Check sheet for the modelled part. Datum: model origin and axes. Units: mm. Round coordinates to 2 decimals unless told otherwise and drop trailing zeros. Loops run counter-clockwise (first coordinate to the right, second up) from the corner with the lowest first, then second, coordinate; pieces in that order, holes last. Notation, with made-up numbers: (-24.75, 42) -> (4.25, 42) arc R18 cw to (4.25, 61) -> close; hole circle Ø9 at (21, -9). An arc over 180 degrees is marked (long way). Return JSON: item names as keys, results as strings.
Autodesk Inventor part; units mm, degrees
ref_plane "YZ Plane" through (0, 0, 0) normal (1, 0, 0) x (0, 1, 0)
ref_plane "XZ Plane" through (0, 0, 0) normal (0, 1, 0) x (-1, 0, 0)
ref_plane "XY Plane" through (0, 0, 0) normal (0, 0, 1) x (1, 0, 0)
sketch "スケッチ3" plane through (0, 0, 0) normal (0, 0, 1) x (1, 0, 0)
  line L0 (60, -99.3436) -> (-60, -99.3436)
  line L1 (-60, -99.3436) -> (-60, 99.3436)
  line L2 (-60, 99.3436) -> (60, 99.3436)
  line L3 (60, 99.3436) -> (60, -99.3436)
  line L4 (60, -99.3436) -> (-60, 99.3436) construction
  line L5 (-60, -99.3436) -> (60, 99.3436) construction
  point P0 (0, 0)
  dimension "d25" = 120
extrude "押し出し1" add sketch "スケッチ3" against normal blind 3
sketch "スケッチ4" plane through (0, 0, 0) normal (0, 0, 1) x (1, 0, 0)
  line L0 (0, 45.0711) -> (68.3595, 45.0711)
  line L1 (68.3595, 45.0711) -> (-74.3824, 45.0711)
  line L2 (-74.3824, 45.0711) -> (108.1656, 45.0711)
  line L3 (108.1656, 45.0711) -> (108.1656, 129.4154)
  line L4 (108.1656, 129.4154) -> (-74.3824, 129.4154)
  line L5 (-74.3824, 129.4154) -> (-74.3824, 45.0711)
  point P0 (0, 0)
extrude "押し出し4" cut sketch "スケッチ4" against normal blind 10
sketch "スケッチ12" plane through (0, 0, 0) normal (0, 0, 1) x (1, 0, 0)
  circle A0 centre (0, 0) radius 9
  circle A1 centre (0, 0) radius 22.5
  dimension "d85" = 18
  dimension "d93" = 45
sketch "スケッチ13" plane through (0, 0, 0) normal (0, 0, 1) x (1, 0, 0)
  circle A0 centre (0, 0) radius 7.5
  circle A1 centre (0, 0) radius 32.5
  circle A2 centre (31.7707, 6.8465) radius 25
  circle A3 centre (31.7707, 6.8465) radius 7.5
  circle A4 centre (31.7707, 6.8465) radius 32.5
  circle A5 centre (28.5436, -25.4929) radius 25
  circle A6 centre (28.5436, -25.4929) radius 20
  circle A7 centre (28.5436, -25.4929) radius 60
  circle A8 centre (0, -78.2685) radius 40
  circle A9 centre (0, -78.2685) radius 50
  circle A10 centre (31.7707, 6.8465) radius 5.05
  circle A11 centre (28.5436, -25.4929) radius 9.55
  circle A12 centre (0, -78.2685) radius 9.55
  dimension "d87" = 65
  dimension "d89" = 65
  dimension "d91" = 120
  dimension "d86" = 15
  dimension "d88" = 15
  dimension "d90" = 40
  dimension "d92" = 100
  dimension "d96" = 10.1
  dimension "d97" = 19.1
  dimension "d98" = 19.1
extrude "押し出し15" cut sketch "スケッチ12" against normal blind 10 contours A0
extrude "押し出し16" cut sketch "スケッチ13" against normal blind 10 contours A10 A1 | A1 A10 | A11 A1 A2 | A2 A1 A4 A11 | A4 A1 A11 | A2 A11 A4 A1 | A1 A11 A2 | A4 A11 A1 | A12 A7 | A7 A12
sketch "スケッチ14" plane through (0, 0, 0) normal (0, 0, 1) x (1, 0, 0)
  line L0 (-60, -99.3436) -> (-60, 45.0711)
  line L1 (60, 45.0711) -> (60, -99.3436)
  line L2 (-60, 45.0711) -> (60, 45.0711)
  line L3 (60, 45.0711) -> (60, -92.9289)
  line L4 (60, -92.9289) -> (-60, -92.9289)
  line L5 (-60, -92.9289) -> (-60, 45.0711)
  point P0 (0, 0)
  dimension "d101" = 138
extrude "押し出し17" cut sketch "スケッチ14" against normal blind 10 keep common part
sketch "スケッチ15" plane through (-60, 45.0711, 0) normal (0, 1, 0) x (1, 0, 0)
  line L0 (-15.5399, 21.7204) -> (138.9638, 21.7204)
  line L1 (138.9638, 21.7204) -> (138.9638, -41.1938)
  line L2 (138.9638, -41.1938) -> (-15.5399, -41.1938)
  line L3 (-15.5399, -41.1938) -> (-15.5399, 21.7204)
  point P0 (60, 0)
extrude "押し出し18" cut sketch "スケッチ15" against normal blind 10
sketch "スケッチ16" plane through (0, 0, 0) normal (0, 0, 1) x (1, 0, 0)
  circle A0 centre (31.7707, 6.8465) radius 5.05
  circle A1 centre (31.7707, 6.8465) radius 25
  circle A2 centre (28.5436, -25.4929) radius 9.55
  circle A3 centre (28.5436, -25.4929) radius 25
  circle A4 centre (55, -13) radius 2.1
  circle A5 centre (-55, -13) radius 2.1
  circle A6 centre (0, 29) radius 2.1
  point P0 (0, 0)
  dimension "d109" = 50
  dimension "d110" = 50
  dimension "d111" = 4.2
  dimension "d112" = 4.2
  dimension "d113" = 4.2
extrude "押し出し19" cut sketch "スケッチ16" against normal blind 10 contours A4 | A5 | A6
sketch "スケッチ17" plane through (0, 0, 0) normal (0, 0, 1) x (1, 0, 0)
  line L0 (0, 0) -> (0, 14.5)
  line L1 (0, 14.5) -> (0, -14.5)
  circle A0 centre (0, 14.5) radius 2.15
  circle A1 centre (0, -14.5) radius 2.15
  dimension "d116" = 14.5
  dimension "d117" = 29
  dimension "d118" = 4.3
  dimension "d119" = 4.3
extrude "押し出し20" cut sketch "スケッチ17" against normal blind 10
sketch "スケッチ18" plane through (0, 0, 0) normal (0, 0, 1) x (1, 0, 0)
  circle A0 centre (-52.5, -85.929) radius 1.6
  circle A1 centre (-52.5, -77.929) radius 1.6
  circle A2 centre (52.5, -77.929) radius 1.6
  circle A3 centre (52.5, -85.929) radius 1.6
  point P0 (0, 0)
  dimension "d122" = 3.2
  dimension "d123" = 3.2
  dimension "d124" = 3.2
  dimension "d125" = 3.2
extrude "押し出し21" cut sketch "スケッチ18" against normal blind 3.2
fillet "フィレット2" radius 2 4 edges at (-60, 35.0711, -1.5) (60, 35.0711, -1.5) (60, -92.9289, -1.5) (-60, -92.9289, -1.5)
properties part number "板2" material "アルミニウム 6061"
Q1. Material ranges on line 1 (Y direction, x = 52.5, z = -2.4); line 2 (X direction, y = -14.5, z = -2.05); line 3 (Y direction, x = -55, z = -0.9), recorded low to high.
Results list:
{"line 1": "-92.93 to -87.53, -84.33 to -79.53, -76.33 to 35.07", "line 2": "-60 to -56.47, -53.53 to -2.15, 2.15 to 53.53, 56.47 to 60", "line 3": "-92.93 to -15.1, -10.9 to 35.07"}
Q2. Section check B-B (x = 23.5). Record the boundary of the cut face in (y, z), then the cut area to 3 significant figures.
Results list:
{"outline": "(-92.93, -3) -> (-33.6, -3) -> (-33.6, 0) -> (-92.93, 0) -> close; (-17.38, -3) -> (35.07, -3) -> (35.07, 0) -> (-17.38, 0) -> close", "area": "335 mm^2"}
Q3. Go/stop test with a flat-tipped pin: pin 1 (5 mm diameter, centred on x = 55, y = -13, fed in from +Z). Record where the tip stops, or that it passes through.
Results list:
{"pin 1": "z = 0"}
Q4. Section check A-A (x = 5). Record the boundary of the cut face in (y, z) (3 decimals).
Results list:
{"outline": "(-92.929, -3) -> (-86.405, -3) -> (-86.405, 0) -> (-92.929, 0) -> close; (-70.132, -3) -> (-7.483, -3) -> (-7.483, 0) -> (-70.132, 0) -> close; (7.483, -3) -> (35.071, -3) -> (35.071, 0) -> (7.483, 0) -> close"}
Q5. Section check C-C (z = -0.75). Count the separate pieces of the cut face and the enclosed holes in it, then the cut area to 3 significant figures.
Results list:
{"separate pieces": "1", "enclosed holes": "13", "area": "14,300 mm^2"}
Q6. Draft check along X on faces 1 (the flat face through (60, -28, -1)), 2 (the flat face through (-60, -30, -1)), 3 (the cylindrical face through (57.003, -12.369, -1.479)). Enter one of: released by +X, released by -X, zero draft, split by the parting line, or undercut.
Results list:
{"face 1": "released by +X", "face 2": "released by -X", "face 3": "undercut"}
